Check sheet for the modelled part. Datum: model origin and axes. Units: mm. A direction names the side the tool comes from. Give positions to 0.01 mm unless a question says otherwise; leave off trailing zeros. Loops run counter-clockwise (first coordinate to the right, second up) from the corner with the lowest first, then second, coordinate; pieces in that order, holes last. Notation, with made-up numbers: (17.5, -3) -> (42.5, -3) arc R12 cw to (42.5, 4) -> close; hole circle Ø7 at (-1.5, 67.25). An arc over 180 degrees is marked (long way). Write each question's results on one line, items separated by ' | '. Start each with the question number.
1. Material ranges on L1, parallel to X at y = -4.5, z = 58; L2, parallel to X at y = 7.1, z = 88, recorded low to high. Write a range as from..to.
2. Gauge pin test, flat ends, axial feed: pin 1 Ø2.5 at (x, z) = (0, 88) entering from -Y; pin 2 Ø5 at (x, z) = (0, 190) entering from -Y; pin 3 Ø5 at (x, z) = (0, 175) entering from +Y. Record the tip position at first contact, or that the pin passes through.
3. Cross-section at A-A on y = 0.25. Record the boundary of the cut face in (x, z), and give its area (3 significant figures).
4. Tool access check on faces 1 (the face through (-0.867, 7.007, 91.905)), 2 (the face through (-7, 0, 0)), 3 (the face through (1.201, -7.007, 186.185)), 4 (the face through (0, -6.5, 123)). Record the directions out of +Z, -Z, +X, -X, +Y, -Y that give a thin tool (end or side, any length) a straight path to the whole face; none if there is none.
5. Mould release check, pull along X, two halves, no side actions. Record for faces 5 (the face through (1.201, 7.007, 208.815)), 6 (the face through (7.5, 0, 123)), 7 (the face through (-7.5, 0, 123)): +X half, -X half, draft (parallel to the pull), parting line (faces both ways), or undercut.
6. Cross-section at B-B on z = 25.5. Record the boundary of the cut face in (x, y).
from build123d import *

# Parameters (mm, degrees)
SKETCH_1_W          = 15
SKETCH_1_H          = 15
SKETCH_1_W_2        = 13
SKETCH_1_H_2        = 13
EXTRUDE_1_DEPTH     = 250
SKETCH_2_R          = 1.5
CUT_EXTRUDE_1_DEPTH = 250
SKETCH_3_R          = 4
CUT_EXTRUDE_2_DEPTH = 1.5
SKETCH_4_R          = 4
CUT_EXTRUDE_3_DEPTH = 1.5


with BuildPart() as part:
    # Sketch 1 → Extrude 1 (new body)
    with BuildSketch(Plane.XY):
        Rectangle(SKETCH_1_W, SKETCH_1_H)
        Rectangle(SKETCH_1_W_2, SKETCH_1_H_2, mode=Mode.SUBTRACT)
    extrude(amount=EXTRUDE_1_DEPTH)

    # Sketch 2 → Cut-Extrude 1 (cut)
    with BuildSketch(Plane(origin=(0, 7.5, 0), x_dir=(1, 0, 0), z_dir=(0, 1, 0))):
        with Locations(Location((0, -218, 0), (0, 0, 270))):
            Circle(SKETCH_2_R)
        with Locations(Location((0, -205, 0), (0, 0, 270))):
            Circle(SKETCH_2_R)
        with Locations(Location((0, -175, 0), (0, 0, 270))):
            Circle(SKETCH_2_R)
        with Locations(Location((0, -162, 0), (0, 0, 270))):
            Circle(SKETCH_2_R)
        with Locations(Location((0, -190, 0), (0, 0, 270))):
            Circle(SKETCH_2_R)
        with Locations((0, -60)):
            Circle(SKETCH_2_R)
        with Locations((0, -88)):
            Circle(SKETCH_2_R)
        with Locations((0, -75)):
            Circle(SKETCH_2_R)
        with Locations((0, -45)):
            Circle(SKETCH_2_R)
        with Locations((0, -32)):
            Circle(SKETCH_2_R)
    extrude(amount=-CUT_EXTRUDE_1_DEPTH, mode=Mode.SUBTRACT)

    # Sketch 3 → Cut-Extrude 2 (cut)
    with BuildSketch(Plane(origin=(0, 7.5, 0), x_dir=(1, 0, 0), z_dir=(0, 1, 0))):
        with Locations(Location((0, -218, 0), (0, 0, 270))):
            Circle(SKETCH_3_R)
        with Locations(Location((0, -205, 0), (0, 0, 270))):
            Circle(SKETCH_3_R)
        with Locations((0, -75)):
            Circle(SKETCH_3_R)
        with Locations(Location((0, -162, 0), (0, 0, 270))):
            Circle(SKETCH_3_R)
        with Locations(Location((0, -175, 0), (0, 0, 270))):
            Circle(SKETCH_3_R)
        with Locations((0, -88)):
            Circle(SKETCH_3_R)
        with Locations((0, -45)):
            Circle(SKETCH_3_R)
        with Locations((0, -32)):
            Circle(SKETCH_3_R)
    extrude(amount=-CUT_EXTRUDE_2_DEPTH, mode=Mode.SUBTRACT)

    # Sketch 4 → Cut-Extrude 3 (cut)
    with BuildSketch(Plane.XZ.offset(7.5)):
        with Locations(Location((0, 60, 0), (0, 0, 270))):
            Circle(SKETCH_4_R)
        with Locations(Location((0, 190, 0), (0, 0, 270))):
            Circle(SKETCH_4_R)
    extrude(amount=-CUT_EXTRUDE_3_DEPTH, mode=Mode.SUBTRACT)


solid = part.part
Geometry says:
1) L1: -7.5..-6.5, 6.5..7.5 | L2: -7.5..-4, 4..7.5
2) pin 1: through | pin 2: y = 6.5 | pin 3: y = -6.5
3) outline: (-7.5, 0) -> (-6.5, 0) -> (-6.5, 250) -> (-7.5, 250) -> close; (6.5, 0) -> (7.5, 0) -> (7.5, 250) -> (6.5, 250) -> close | area: 500 mm^2
4) face 1: +Y | face 2: -Z, +X, -X, +Y, -Y | face 3: -Y | face 4: +Z, -Z
5) face 5: undercut | face 6: +X half | face 7: -X half
6) outline: (-7.5, -7.5) -> (7.5, -7.5) -> (7.5, 7.5) -> (-7.5, 7.5) -> close; hole (-6.5, -6.5) -> (6.5, -6.5) -> (6.5, 6.5) -> (-6.5, 6.5) -> close
